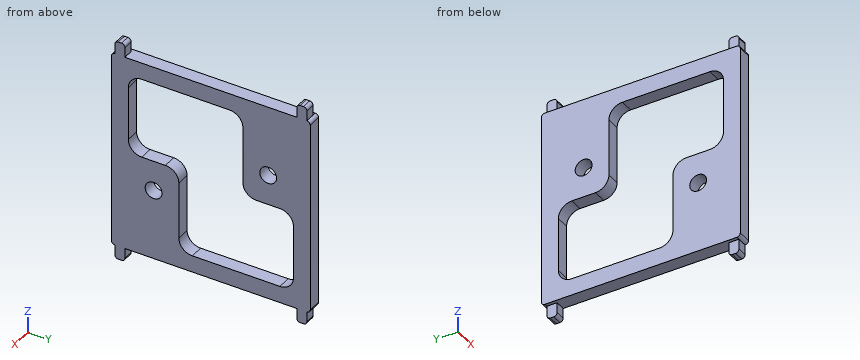
```python
from build123d import *

# Parameters (mm, degrees)
F0_W     = 3
F0_H     = 4
F0_W_2   = 15
F0_H_2   = 25
F0_R     = 2.5
F1_DEPTH = 4
F2_W     = 3
F2_H     = 4
F3_DEPTH = 1
F4_R     = 4
F5_R     = 0.99999


# Not quite as in the source:
# - a fillet or chamfer is up to 0.001 mm smaller than in the source, because OpenCascade refuses the exact size


with BuildPart() as f1:
    # F0 (on Right) → F1 (new body)
    with BuildSketch(Plane.YZ):
        Polygon((-28.5, 29.5), (-29.5, 29.5), (-29.5, -29.5), (-28.5, -29.5), (-25.5, -29.5), (25.5, -29.5), (28.5, -29.5), (29.5, -29.5), (29.5, 29.5), (28.5, 29.5), (25.5, 29.5), (-25.5, 29.5), align=None)
        Polygon((-24.5, 0.5), (-24.5, 24.5), (9.5, 24.5), (24.5, 24.5), (24.5, -0.5), (24.5, -24.5), (-9.5, -24.5), (-24.5, -24.5), align=None, mode=Mode.SUBTRACT)
        with Locations((-27, 31.5)):
            Rectangle(F0_W, F0_H)
        with Locations((27, 31.5)):
            Rectangle(F0_W, F0_H)
        with Locations((-27, -31.5)):
            Rectangle(F0_W, F0_H)
        with Locations((27, -31.5)):
            Rectangle(F0_W, F0_H)
        with Locations((-17, -12)):
            Rectangle(F0_W_2, F0_H_2)
        with Locations((-17, -8.5)):
            Circle(F0_R, mode=Mode.SUBTRACT)
        with Locations((17, 12)):
            Rectangle(F0_W_2, F0_H_2)
        with Locations((17, 8.5)):
            Circle(F0_R, mode=Mode.SUBTRACT)
    extrude(amount=F1_DEPTH)

    # F2 (on face) → F3 (cut)
    with BuildSketch(Plane(origin=(0, 0, 0), x_dir=(0, -1, 0), z_dir=(-1, 0, 0))):
        with Locations((-27, 31.5)):
            Rectangle(F2_W, F2_H)
        with Locations((27, 31.5)):
            Rectangle(F2_W, F2_H)
        with Locations((-27, -31.5)):
            Rectangle(F2_W, F2_H)
        with Locations((27, -31.5)):
            Rectangle(F2_W, F2_H)
    extrude(amount=-F3_DEPTH, mode=Mode.SUBTRACT)

    # F4
    f4_edges = [f1.edges().sort_by_distance(p)[0] for p in [
        (2, 9.5, -0.5),
        (2, 9.5, 24.5),
        (2, 24.5, -0.5),
        (2, -9.5, 0.5),
        (2, -24.5, 0.5),
        (2, -9.5, -24.5),
        (2, -24.5, 24.5),
        (2, 24.5, -24.5),
    ]]
    fillet(f4_edges, radius=F4_R)

    # F5 (radius 1 in the source; OpenCascade refuses exactly that, so slightly less here)
    f5_edges = [f1.edges().sort_by_distance(p)[0] for p in [
        (2.5, 28.5, 33.5),
        (2.5, 25.5, 33.5),
        (2.5, -25.5, 33.5),
        (2.5, -28.5, 33.5),
        (2, 29.5, 29.5),
        (2, -29.5, 29.5),
        (2, -29.5, -29.5),
        (2.5, -28.5, -33.5),
        (2.5, -25.5, -33.5),
        (2, 29.5, -29.5),
        (2.5, 28.5, -33.5),
        (2.5, 25.5, -33.5),
    ]]
    fillet(f5_edges, radius=F5_R)


solid = f1.part
```
Check sheet for the modelled part. Datum: model origin and axes. Units: mm. Give positions to 0.01 mm unless a question says otherwise; leave off trailing zeros. Loops run counter-clockwise (first coordinate to the right, second up) from the corner with the lowest first, then second, coordinate; pieces in that order, holes last. Notation, with made-up numbers: M 57,15 L 104,15 A5 cw 104,24 Z; hole C -12,57 d2. An arc over 180 degrees is marked long. Answer in a Markdown table with one row per item.
1) Cross-section at D-D (z = -14.5). Enter the section's corners in (x, y), plus the area to 3 significant figures.
Solutions:
| item | result |
|---|---|
| outline | M 0,-29.5 L 4,-29.5 L 4,-9.5 L 0,-9.5 Z; M 0,24.5 L 4,24.5 L 4,29.5 L 0,29.5 Z |
| area | 100 mm^2 |
2) Cross-section at C-C (y = 17). Enter the section's corners in (x, z).
Solutions:
| item | result |
|---|---|
| outline | M 0,-29.5 L 4,-29.5 L 4,-24.5 L 0,-24.5 Z; M 0,-0.5 L 4,-0.5 L 4,6 L 0,6 Z; M 0,11 L 4,11 L 4,29.5 L 0,29.5 Z |
3) Cross-section at A-A (y = 2). Enter the section's corners in (x, z).
Solutions:
| item | result |
|---|---|
| outline | M 0,-29.5 L 4,-29.5 L 4,-24.5 L 0,-24.5 Z; M 0,24.5 L 4,24.5 L 4,29.5 L 0,29.5 Z |
4) Thickness scan on line 1 (Z direction, x = 2, y = -17); line 2 (Y direction, x = 3.5, z = 15.5); line 3 (Z direction, x = 0.3, y = 5). Record the ranges inside material, lowest first.
Solutions:
| item | result |
|---|---|
| line 1 | z = -29.5 to -11, -6 to 0.5, 24.5 to 29.5 |
| line 2 | y = -29.5 to -24.5, 9.5 to 29.5 |
| line 3 | z = -29.5 to -24.5, 24.5 to 29.5 |
5) Depth check by flat-ended pin: pin 1 (0.9 mm diameter, centred on x = 2, z = -31.5, fed in from -Y); pin 2 (12 mm diameter, centred on y = 6, z = -3.5, fed in from +X); pin 3 (1.2 mm diameter, centred on x = 2, y = -16, fed in from +Z); pin 4 (1.5 mm diameter, centred on y = 26.5, z = -31.5, fed in from -X). Enter the tip coordinate at first touch or a pass-through.
Solutions:
| item | result |
|---|---|
| pin 1 | stops at y = -28.5 |
| pin 2 | passes through |
| pin 3 | stops at z = 29.5 |
| pin 4 | stops at x = 1 |
6) Cross-section at B-B (z = 8.5). Enter the section's corners in (x, y).
Solutions:
| item | result |
|---|---|
| outline | M 0,-29.5 L 4,-29.5 L 4,-24.5 L 0,-24.5 Z; M 0,9.5 L 4,9.5 L 4,14.5 L 0,14.5 Z; M 0,19.5 L 4,19.5 L 4,29.5 L 0,29.5 Z |
